Autodesk Inventor part; units mm, degrees
ref_plane "YZ Plane" through (0, 0, 0) normal (1, 0, 0) x (0, 1, 0)
ref_plane "XZ Plane" through (0, 0, 0) normal (0, 1, 0) x (-1, 0, 0)
ref_plane "XY Plane" through (0, 0, 0) normal (0, 0, 1) x (1, 0, 0)
sketch "Sketch1" plane through (0, 0, 0) normal (0, 1, 0) x (-1, 0, 0)
  circle A0 centre (0, 0) radius 7.1045
  dimension "d0" = 14.209
extrude "Extrusion1" add sketch "Sketch1" along normal blind 4
sketch "Sketch2" plane through (0, 4, 0) normal (0, 1, 0) x (1, 0, 0)
  circle A0 centre (0, 0) radius 7.1045
  circle A1 centre (0, 0) radius 3.5
  circle A2 centre (0, 0) radius 2
  dimension "d3" = 7
  dimension "d4" = 4
extrude "Extrusion2" add sketch "Sketch2" along normal blind 6 contours A1
properties part number "ozubene_kolecko_otaceni_ramene_male"
Read the model definition and answer for the solid it produces. Units are mm, in the model's axes. A direction names the side the tool comes from. Round coordinates to 2 decimals unless told otherwise and drop trailing zeros. Write each loop counter-clockwise with the first axis right and the second up, starting at its lowest first coordinate (ties: lowest second). Pieces come first, ordered by that corner, then holes. Notation, with made-up numbers: (-8, 77) - (18, 77) arc R30 ccw to (18, 101) - close; hole circle Ø10 at (-30.5, 68.5). An arc over 180 degrees is marked (long way). Use a Markdown table: item, result.
(1) The part is cut by section D-D (y = 3.75). Write down the section's boundary in (x, z), then the cut area to 3 significant figures.
Reported:
| item | result |
|---|---|
| outline | circle Ø14.21 at (0, 0) |
| area | 159 mm2 |
(2) The part is cut by section C-C (y = 7.5). Write down the section's boundary in (x, z), then the cut area to 3 significant figures.
Reported:
| item | result |
|---|---|
| outline | circle Ø7 at (0, 0); hole circle Ø4 at (0, 0) |
| area | 25.9 mm2 |
(3) Which of the six approach directions +Z, -Z, +X, -X, +Y, -Y give full straight-line access (tool end or side, diameter ignored) to faces 1 (the flat face through (0, 4, 0)), 2 (the flat face through (2, 10, 2))?
Reported:
| item | result |
|---|---|
| face 1 | +Y |
| face 2 | +Z, -Z, +X, -X, +Y |
(4) The mould has two halves that part along X. Classify faces 3 (the flat face through (3.3, 4, 1.7)), 4 (the cylindrical face through (0, 7, -2)), 5 (the cylindrical face through (3.233, 6.958, -1.341)): released by +X, released by -X, zero draft, split by the parting line, or undercut.
Reported:
| item | result |
|---|---|
| face 3 | zero draft |
| face 4 | undercut |
| face 5 | split by the parting line |
(5) Straight lines are drawn through the part: line 1 along Z through (x, y) = (0, 7.5); line 2 along Y through (x, z) = (4.5, -2.25). For each, find the intervals that lie inside material, in ascending order. Write a range as [from, to].
Reported:
| item | result |
|---|---|
| line 1 | [-3.5, -2], [2, 3.5] |
| line 2 | [0, 4] |
(6) The part is cut by section B-B (x = 0). Write down the section's boundary in (y, z).
Reported:
| item | result |
|---|---|
| outline | (0, -7.1) - (4, -7.1) - (4, -3.5) - (10, -3.5) - (10, -2) - (4, -2) - (4, 2) - (10, 2) - (10, 3.5) - (4, 3.5) - (4, 7.1) - (0, 7.1) - close |
(7) The part is cut by section A-A (z = 0). Write down the section's boundary in (x, y).
Reported:
| item | result |
|---|---|
| outline | (-7.1, 0) - (7.1, 0) - (7.1, 4) - (3.5, 4) - (3.5, 10) - (2, 10) - (2, 4) - (-2, 4) - (-2, 10) - (-3.5, 10) - (-3.5, 4) - (-7.1, 4) - close |
(8) Each of these flat-tipped pins is pushed along its axis until it touches: pin 1 Ø1 at (y, z) = (1, 5.5) entering from -X; pin 2 Ø1.5 at (x, y) = (-5.5, 7) entering from -Z; pin 3 Ø1 at (x, y) = (0, 8) entering from -Z; pin 4 Ø6 at (y, z) = (1.5, -3.5) entering from +X. Where does it stop, or does it pass through?
Reported:
| item | result |
|---|---|
| pin 1 | x = -5.05 |
| pin 2 | through |
| pin 3 | z = -3.5 |
| pin 4 | x = 7.09 |
